from build123d import *

# Parameters (mm, degrees)
SKETCH2_W = 0.3
SKETCH2_H = 8


with BuildPart() as part:
    # Sketch3 → Revolve1 (revolve)
    with BuildSketch(Plane.XY, mode=Mode.PRIVATE) as revolve1_sk:
        Polygon((0.9, 2.676607812), (1.05, 2.676607812), (1.05, 3.240637489), (1.96196636, 2.328671129), (1.96196636, -3.923392188), (1.838146931, -3.923392188), (1.838146931, 2.328671129), align=None)
    revolve(revolve1_sk.sketch.rotate(Axis((0, 19.759006236, 0), (0, -1, 0)), 90), axis=Axis((0, 19.759006236, 0), (0, -1, 0)))

    # Sketch2 → Revolve2 (revolve)
    with BuildSketch(Plane.XY, mode=Mode.PRIVATE) as revolve2_sk:
        with Locations((0.9, 6.676607812)):
            Rectangle(SKETCH2_W, SKETCH2_H)
    revolve(revolve2_sk.sketch.rotate(Axis((0, 19.759006236, 0), (0, -1, 0)), 90), axis=Axis((0, 19.759006236, 0), (0, -1, 0)))


solid = part.part
Check sheet for the modelled part. Datum: model origin and axes. Units: mm. Round coordinates to 2 decimals unless told otherwise and drop trailing zeros. Write each loop counter-clockwise with the first axis right and the second up, starting at its lowest first coordinate (ties: lowest second). Pieces come first, ordered by that corner, then holes. Notation, with made-up numbers: (75.5, 11.25) - (129.5, 11.25) arc R22 ccw to (129.5, 39.25) - close; hole circle Ø2 at (6.5, 76). An arc over 180 degrees is marked (long way). Return JSON: item names as keys, results as strings.
Q1. Draft check along Z on faces 1 (the cylindrical face through (-0.32, 7.01, 1)), 2 (the cylindrical face through (-0.225, 6.733, 0.715)). Enter one of: released by +Z, released by -Z, zero draft, split by the parting line, or undercut.
Returned:
{"face 1": "split by the parting line", "face 2": "undercut"}
Q2. Cross-section at B-B (z = 0). Record the boundary of the cut face in (x, y), then the cut area to 3 significant figures.
Returned:
{"outline": "(-1.96, -3.92) - (-1.84, -3.92) - (-1.84, 2.33) - (-0.9, 2.68) - (-0.75, 2.68) - (-0.75, 10.68) - (-1.05, 10.68) - (-1.05, 3.24) - (-1.96, 2.33) - close; (0.75, 2.68) - (0.9, 2.68) - (1.84, 2.33) - (1.84, -3.92) - (1.96, -3.92) - (1.96, 2.33) - (1.05, 3.24) - (1.05, 10.68) - (0.75, 10.68) - close", "area": "6.96 mm²"}
Q3. Depth check by flat-ended pin: P1, Ø1, axis at y = 4.5, z = 1, coming from the +X side; P2, Ø1.5, axis at x = -0.5, y = 2, coming from the +Z side; P3, Ø1.7, axis at x = 0, z = 0, coming from the -Y side; P4, Ø1.5, axis at x = -1, y = -1, coming from the -Z side. Enter the tip coordinate at first touch or a pass-through.
Returned:
{"P1": "stops at x = 0.92", "P2": "stops at z = 1.96", "P3": "stops at y = 2.68", "P4": "stops at z = -1.95"}
Q4. Cross-section at D-D (y = 6.75). Record the boundary of the cut face in (x, z), then the cut area to 3 significant figures.
Returned:
{"outline": "circle Ø2.1 at (0, 0); hole circle Ø1.5 at (0, 0)", "area": "1.70 mm²"}
Q5. Cross-section at A-A (x = 0). Record the boundary of the cut face in (y, z).
Returned:
{"outline": "(-3.92, -1.96) - (2.33, -1.96) - (3.24, -1.05) - (10.68, -1.05) - (10.68, -0.75) - (2.68, -0.75) - (2.68, -0.9) - (2.33, -1.84) - (-3.92, -1.84) - close; (-3.92, 1.84) - (2.33, 1.84) - (2.68, 0.9) - (2.68, 0.75) - (10.68, 0.75) - (10.68, 1.05) - (3.24, 1.05) - (2.33, 1.96) - (-3.92, 1.96) - close"}
Q6. Scan lines: L1, parallel to X at y = 7.5, z = 0; L2, parallel to Z at x = -1.4, y = -2; L3, parallel to Z at x = -0.35, y = 4. Record each from-to range of solid material in increasing order. Write a range as from..to.
Returned:
{"L1": "x = -1.05..-0.75, 0.75..1.05", "L2": "z = -1.37..-1.19, 1.19..1.37", "L3": "z = -0.99..-0.66, 0.66..0.99"}
Q7. Cross-section at C-C (y = -2). Record the boundary of the cut face in (x, z), then the cut area to 3 significant figures.
Returned:
{"outline": "circle Ø3.92 at (0, 0); hole circle Ø3.68 at (0, 0)", "area": "1.48 mm²"}
